from build123d import *

# Parameters (mm, degrees)
SKETCH1_W           = 22.225
SKETCH1_H           = 152.4
BOSS_EXTRUDE1_DEPTH = 31.75
SKETCH2_W           = 1.5875
SKETCH2_H           = 30.1625
CUT_EXTRUDE1_DEPTH  = 23.225
SKETCH3_W           = 1.5875
SKETCH3_H           = 14.2875
BOSS_EXTRUDE2_DEPTH = 22.225


with BuildPart() as part:
    # Sketch1 → Boss-Extrude1 (new body)
    with BuildSketch(Plane(origin=(0, 0, 0), x_dir=(1, 0, 0), z_dir=(0, 1, 0))):
        with Locations((11.1125, 76.2)):
            Rectangle(SKETCH1_W, SKETCH1_H)
    extrude(amount=BOSS_EXTRUDE1_DEPTH)

    # Sketch2 → Cut-Extrude1 (cut, through all)
    with BuildSketch(Plane(origin=(22.225, 0, 0), x_dir=(0, 0, -1), z_dir=(1, 0, 0))):
        with Locations((0.79375, 15.08125)):
            Rectangle(SKETCH2_W, SKETCH2_H)
    extrude(amount=-CUT_EXTRUDE1_DEPTH, mode=Mode.SUBTRACT)

    # Sketch3 → Boss-Extrude2 (add)
    with BuildSketch(Plane(origin=(22.225, 0, 0), x_dir=(0, 0, -1), z_dir=(1, 0, 0))):
        with Locations((153.19375, 7.14375)):
            Rectangle(SKETCH3_W, SKETCH3_H)
    extrude(amount=-BOSS_EXTRUDE2_DEPTH)


solid = part.part
Build history of the part. All positions in model axes, mm. A direction names the side the tool comes from. Coordinates: 2 decimals unless noted, no trailing zeros. Order: outer loops, then holes, each group sorted by start corner. A loop starts at its lowest first (then second) coordinate and runs counter-clockwise, first axis right, second up. Notation, with made-up numbers: (54.25, 75.25) - (94.25, 75.25) arc R10 cw to (94.25, 91.25) - close; hole circle Ø7 at (87, 2). An arc over 180 degrees is marked (long way). Write each question's results on one line, items separated by ' | '. Start each with the question number.
Item 1: Band-saw the part on B-B on y = 18. Write the cut outline in (x, z) (1 decimal), and give its area (3 significant figures).
Item 2: Tool access for faces 1 (the face through (11, 23, -152.4)), 2 (the face through (11, 31.75, -77)), 3 (the face through (11, 15, -1.588)): list every direction of +Z, -Z, +X, -X, +Y, -Y with a clear straight run to the whole face (end or side of a thin tool).
Item 3: Flat gauge pins, fed straight in: pin 1 (8.5 mm diameter, centred on x = 10, y = 20.5, fed in from -Z); pin 2 (6.5 mm diameter, centred on x = 15.5, y = 17, fed in from +Z); pin 3 (1.7 mm diameter, centred on x = 8.5, z = -0.5, fed in from -Y). Where does each tip first touch, or does it go through?
Item 4: Band-saw the part on A-A on x = 18.75. Write the cut outline in (y, z).
Item 5: Wall check: probe 1 along Z at (x, y) = (13.75, 19); probe 2 along Z at (x, y) = (14.5, 2.5). Give the ranges that are in metal, low to high. Write a range as [from, to].
Numbers:
1) outline: (0, -152.4) - (22.2, -152.4) - (22.2, -1.6) - (0, -1.6) - close | area: 3,350 mm^2
2) face 1: -Z, +X, -X, +Y | face 2: +Z, -Z, +X, -X, +Y | face 3: +Z, +X, -X, -Y
3) pin 1: z = -152.4 | pin 2: z = -1.59 | pin 3: y = 30.16
4) outline: (0, -153.99) - (14.29, -153.99) - (14.29, -152.4) - (31.75, -152.4) - (31.75, 0) - (30.16, 0) - (30.16, -1.59) - (0, -1.59) - close
5) probe 1: [-152.4, -1.59] | probe 2: [-153.99, -1.59]
